```python
from build123d import *

# Parameters (mm, degrees)
BOSS_EXTRUDE1_DEPTH = 7.5
SKETCH2_W           = 1
SKETCH2_H           = 1
BOSS_EXTRUDE2_DEPTH = 1
SKETCH3_W           = 4
SKETCH3_H           = 5
CUT_EXTRUDE1_DEPTH  = 2
SKETCH4_R           = 1.75
SKETCH4_R_2         = 0.4
CUT_EXTRUDE2_DEPTH  = 2
CUT_EXTRUDE3_DEPTH  = 0.5
CHAMFER1_SIZE       = 0.3


with BuildPart() as part:
    # Sketch1 → Boss-Extrude1 (new body, symmetric)
    with BuildSketch(Plane.XY):
        Polygon((-3.75, 0), (3.75, 0), (3.75, 6.8), (1.75, 10), (-2.35, 10), (-3.75, 6.8), align=None)
    extrude(amount=BOSS_EXTRUDE1_DEPTH, both=True)

    # Sketch2 → Boss-Extrude2 (add)
    with BuildSketch(Plane.XZ):
        with Locations((0.45, 5)):
            Rectangle(SKETCH2_W, SKETCH2_H)
        with Locations((0.45, 0)):
            Rectangle(SKETCH2_W, SKETCH2_H)
        with Locations((0.45, -5)):
            Rectangle(SKETCH2_W, SKETCH2_H)
    extrude(amount=BOSS_EXTRUDE2_DEPTH)

    # Sketch3 → Cut-Extrude1 (cut)
    with BuildSketch(Plane(origin=(3.75, 0, 0), x_dir=(0, 0, -1), z_dir=(1, 0, 0))):
        with Locations((-5, 3.4)):
            Rectangle(SKETCH3_W, SKETCH3_H)
        with Locations((0, 3.4)):
            Rectangle(SKETCH3_W, SKETCH3_H)
        with Locations((5, 3.4)):
            Rectangle(SKETCH3_W, SKETCH3_H)
    extrude(amount=-CUT_EXTRUDE1_DEPTH, mode=Mode.SUBTRACT)

    # Sketch4 → Cut-Extrude2 (cut)
    with BuildSketch(Plane(origin=(0, 10, 0), x_dir=(1, 0, 0), z_dir=(0, 1, 0))):
        with Locations((-0.3, 5)):
            Circle(SKETCH4_R)
        with Locations((-0.3, 0)):
            Circle(SKETCH4_R)
        with Locations((-0.3, -5)):
            Circle(SKETCH4_R)
        with Locations((2.45, 2.5)):
            Circle(SKETCH4_R_2)
        with Locations((2.45, -2.5)):
            Circle(SKETCH4_R_2)
        with Locations((-3.05, 2.5)):
            Circle(SKETCH4_R_2)
        with Locations((-3.05, -2.5)):
            Circle(SKETCH4_R_2)
    extrude(amount=-CUT_EXTRUDE2_DEPTH, mode=Mode.SUBTRACT)

    # Sketch5 → Cut-Extrude3 (cut)
    with BuildSketch(Plane(origin=(0, 8, 0), x_dir=(1, 0, 0), z_dir=(0, 1, 0))):
        with BuildLine():
            Line((-1.221836, 1.487521), (-0.3, 0.565685))
            Line((-0.3, 0.565685), (0.124264, 0.989949))
            Line((0.124264, 0.989949), (0.689949, 0.424264))
            Line((0.689949, 0.424264), (0.265685, 0))
            Line((0.265685, 0), (1.187521, -0.921836))
            ThreePointArc((1.187521, -0.921836), (0.937437, -1.237437), (0.621836, -1.487521))
            Line((0.621836, -1.487521), (-0.3, -0.565685))
            Line((-0.3, -0.565685), (-0.724264, -0.989949))
            Line((-0.724264, -0.989949), (-1.289949, -0.424264))
            Line((-1.289949, -0.424264), (-0.865685, 0))
            Line((-0.865685, 0), (-1.787521, 0.921836))
            ThreePointArc((-1.787521, 0.921836), (-1.537437, 1.237437), (-1.221836, 1.487521))
        make_face()
        with BuildLine():
            Line((-1.221836, 6.487521), (-0.3, 5.565685))
            Line((-0.3, 5.565685), (0.124264, 5.989949))
            Line((0.124264, 5.989949), (0.689949, 5.424264))
            Line((0.689949, 5.424264), (0.265685, 5))
            Line((0.265685, 5), (1.187521, 4.078164))
            ThreePointArc((1.187521, 4.078164), (0.937437, 3.762563), (0.621836, 3.512479))
            Line((0.621836, 3.512479), (-0.3, 4.434315))
            Line((-0.3, 4.434315), (-0.724264, 4.010051))
            Line((-0.724264, 4.010051), (-1.289949, 4.575736))
            Line((-1.289949, 4.575736), (-0.865685, 5))
            Line((-0.865685, 5), (-1.787521, 5.921836))
            ThreePointArc((-1.787521, 5.921836), (-1.537437, 6.237437), (-1.221836, 6.487521))
        make_face()
        with BuildLine():
            Line((-1.221836, -3.512479), (-0.3, -4.434315))
            Line((-0.3, -4.434315), (0.124264, -4.010051))
            Line((0.124264, -4.010051), (0.689949, -4.575736))
            Line((0.689949, -4.575736), (0.265685, -5))
            Line((0.265685, -5), (1.187521, -5.921836))
            ThreePointArc((1.187521, -5.921836), (0.937437, -6.237437), (0.621836, -6.487521))
            Line((0.621836, -6.487521), (-0.3, -5.565685))
            Line((-0.3, -5.565685), (-0.724264, -5.989949))
            Line((-0.724264, -5.989949), (-1.289949, -5.424264))
            Line((-1.289949, -5.424264), (-0.865685, -5))
            Line((-0.865685, -5), (-1.787521, -4.078164))
            ThreePointArc((-1.787521, -4.078164), (-1.537437, -3.762563), (-1.221836, -3.512479))
        make_face()
    extrude(amount=-CUT_EXTRUDE3_DEPTH, mode=Mode.SUBTRACT)

    # Chamfer1
    chamfer1_edges = [part.edges().sort_by_distance(p)[0] for p in [
        (3.75, 3.4, 7),
        (3.75, 0.9, 5),
        (3.75, 3.4, 3),
        (3.75, 5.9, 5),
        (3.75, 3.4, 2),
        (3.75, 0.9, 0),
        (3.75, 3.4, -2),
        (3.75, 5.9, 0),
        (3.75, 3.4, -3),
        (3.75, 0.9, -5),
        (3.75, 3.4, -7),
        (3.75, 5.9, -5),
    ]]
    chamfer(chamfer1_edges, length=CHAMFER1_SIZE)


solid = part.part
```
CAD build for the part. Positions are in the model's coordinates, mm. A direction names the side the tool comes from. Coordinates: 2 decimals unless noted, no trailing zeros. Write each loop counter-clockwise with the first axis right and the second up, starting at its lowest first coordinate (ties: lowest second). Pieces come first, ordered by that corner, then holes.
(1) Cut at B-B, the plane z = -2.5. List the corners of the cut face in (x, y) (3 decimals), and give its area (3 significant figures).
(2) Drill centre lines: probe 1 along Z at (x, y) = (-3.05, 8.3); probe 2 along Z at (x, y) = (3, 4.25); probe 3 along Z at (x, y) = (-0.3, 9.1). Where is each one in solid material? Low to high.
(3) Two-plate mould, pull along X, no slides. Class faces 1 (the face through (0.72, 7.754, 5.454)), 2 (the face through (-3.75, 3, 0)), 3 (the face through (3, 8, 0)), 4 (the face through (0.167, 7.754, -3.967)): +X half, -X half, draft (parallel to the pull), parting line (faces both ways), or undercut.
(4) Cut at C-C, the plane y = 9. Count the separate pieces of the cut face and the enclosed holes in it, and give its area (3 significant figures).
(5) Cut at D-D, the plane x = -0.5. List the corners of the cut face in (y, z).
(6) Cut at A-A, the plane y = 1.5. List the corners of the cut face in (x, z), and give its area (3 significant figures).
(7) 3-axis set-ups, long thin cutter, end or side, ignore diameter. For faces 5 (the face through (0.95, -0.5, -5)), 6 (the face through (1.75, 3, -5)), 7 (the face through (-1.32, 7.754, -5.454)), 8 (the face through (0, 5, 7.5)), 9 (the face through (-0.05, -0.5, 5)): which of +Z, -Z, +X, -X, +Y, -Y reach the whole face in a straight line?
(8) Flat gauge pins, fed straight in: pin 1 (0.5 mm diameter, centred on x = 3, z = 0, fed in from +Y); pin 2 (2 mm diameter, centred on x = -1.5, z = -5, fed in from -Y); pin 3 (0.5 mm diameter, centred on x = 0.5, y = -0.5, fed in from +Z); pin 4 (0.8 mm diameter, centred on x = -1.5, z = 1, fed in from +Y). Where does each tip first touch, or does it go through?
Geometry says:
1. outline: (-3.75, 0) - (3.75, 0) - (3.75, 6.8) - (2.85, 8.24) - (2.85, 8) - (2.05, 8) - (2.05, 9.52) - (1.75, 10) - (-2.35, 10) - (-2.65, 9.314) - (-2.65, 8) - (-3.225, 8) - (-3.75, 6.8) - close
1. area: 68.5 mm2
2. probe 1: z = -7.5 to -2.9, -2.1 to 2.1, 2.9 to 7.5
2. probe 2: z = -7.5 to -7, -3 to -2, 2 to 3, 7 to 7.5
2. probe 3: z = -7.5 to -6.75, -3.25 to -1.75, 1.75 to 3.25, 6.75 to 7.5
3. face 1: undercut
3. face 2: -X half
3. face 3: +X half
3. face 4: undercut
4. separate pieces: 1
4. enclosed holes: 3
4. area: 48.1 mm2
5. outline: (0, -7.5) - (10, -7.5) - (10, -6.74) - (8, -6.74) - (8, -5.77) - (7.5, -5.77) - (7.5, -4.23) - (8, -4.23) - (8, -3.26) - (10, -3.26) - (10, -1.74) - (8, -1.74) - (8, -0.77) - (7.5, -0.77) - (7.5, 0.77) - (8, 0.77) - (8, 1.74) - (10, 1.74) - (10, 3.26) - (8, 3.26) - (8, 4.23) - (7.5, 4.23) - (7.5, 5.77) - (8, 5.77) - (8, 6.74) - (10, 6.74) - (10, 7.5) - (0, 7.5) - close
6. outline: (-3.75, -7.5) - (3.75, -7.5) - (3.75, -7.3) - (3.45, -7) - (1.75, -7) - (1.75, -3) - (3.45, -3) - (3.75, -2.7) - (3.75, -2.3) - (3.45, -2) - (1.75, -2) - (1.75, 2) - (3.45, 2) - (3.75, 2.3) - (3.75, 2.7) - (3.45, 3) - (1.75, 3) - (1.75, 7) - (3.45, 7) - (3.75, 7.3) - (3.75, 7.5) - (-3.75, 7.5) - close
6. area: 88.2 mm2
7. face 5: +Z, -Z, +X, -Y
7. face 6: +X
7. face 7: +Y
7. face 8: +Z, +X, -X, +Y, -Y
7. face 9: +Z, -Z, -X, -Y
8. pin 1: stops at y = 8.4
8. pin 2: stops at y = 0
8. pin 3: stops at z = 5.5
8. pin 4: stops at y = 10
